Verification items for the finished model (mm, model axes). Coordinates: 2 decimals unless noted, no trailing zeros. Order: outer loops, then holes, each group sorted by start corner. A loop starts at its lowest first (then second) coordinate and runs counter-clockwise, first axis right, second up. Notation, with made-up numbers: (-4.5, 68.5) - (31.5, 68.5) arc R13 cw to (31.5, 93.5) - close; hole circle Ø10 at (42, 48). An arc over 180 degrees is marked (long way). Answer as CSV lines item,"result". Start each with the question number.
1. Section check B-B (z = 1). Record the cut outline in (x, y) (3 decimals), and give its area (3 significant figures).
2. Section check A-A (x = 33.5). Record the cut outline in (y, z) (3 decimals), and give its area (3 significant figures).
3. Section check C-C (x = 25). Record the cut outline in (y, z).
4. Go/stop test with flat-tipped pins: pin 1 (3.5 mm diameter, centred on x = 16.5, y = 16.5, fed in from +Z); pin 2 (2 mm diameter, centred on x = 16.5, y = 33.5, fed in from -Z). Record where each tip stops, or that it passes through.
5. Material ranges on L1, parallel to Y at x = 16.5, z = 1.15 (3 decimals); L2, parallel to Y at x = 26, z = 0.7, recorded low to high. Write a range as [from, to].
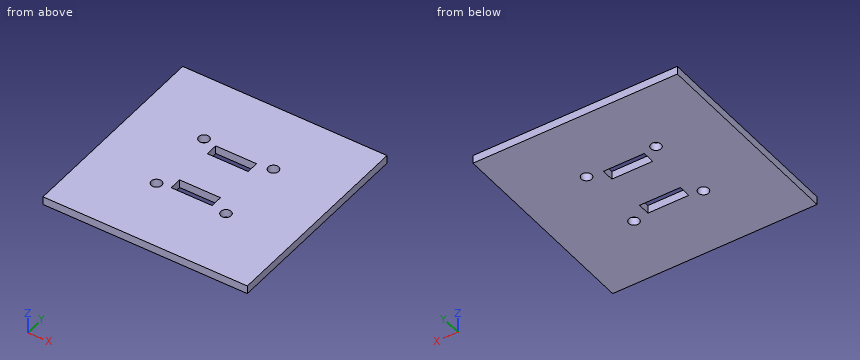
from build123d import *

# Parameters (mm, degrees)
SKETCH1_W           = 50
SKETCH1_H           = 50
BOSS_EXTRUDE1_DEPTH = 2
CUT_EXTRUDE1_REACH  = 72.739
SKETCH3_R           = 1.275
CUT_EXTRUDE2_REACH  = 72.739
SKETCH4_W           = 10
SKETCH4_H           = 3


with BuildPart() as part:
    # Sketch1 → Boss-Extrude1 (new body)
    with BuildSketch(Plane.XY):
        with Locations((25, 25)):
            Rectangle(SKETCH1_W, SKETCH1_H)
    extrude(amount=BOSS_EXTRUDE1_DEPTH)

    # Sketch3 → Cut-Extrude1 (cut, up to next)
    with BuildSketch(Plane.XY.offset(2), mode=Mode.PRIVATE) as cut_extrude1_sk1:
        with Locations((16.5, 33.5)):
            Circle(SKETCH3_R)
    cut_extrude1_tool1 = extrude(cut_extrude1_sk1.sketch, amount=-CUT_EXTRUDE1_REACH, mode=Mode.PRIVATE) & part.part
    # Sketch3 → Cut-Extrude1 (cut, up to next)
    with BuildSketch(Plane.XY.offset(2), mode=Mode.PRIVATE) as cut_extrude1_sk2:
        with Locations((33.5, 33.5)):
            Circle(SKETCH3_R)
    cut_extrude1_tool2 = extrude(cut_extrude1_sk2.sketch, amount=-CUT_EXTRUDE1_REACH, mode=Mode.PRIVATE) & part.part
    # Sketch3 → Cut-Extrude1 (cut, up to next)
    with BuildSketch(Plane.XY.offset(2), mode=Mode.PRIVATE) as cut_extrude1_sk3:
        with Locations((33.5, 16.5)):
            Circle(SKETCH3_R)
    cut_extrude1_tool3 = extrude(cut_extrude1_sk3.sketch, amount=-CUT_EXTRUDE1_REACH, mode=Mode.PRIVATE) & part.part
    # Sketch3 → Cut-Extrude1 (cut, up to next)
    with BuildSketch(Plane.XY.offset(2), mode=Mode.PRIVATE) as cut_extrude1_sk4:
        with Locations((16.5, 16.5)):
            Circle(SKETCH3_R)
    cut_extrude1_tool4 = extrude(cut_extrude1_sk4.sketch, amount=-CUT_EXTRUDE1_REACH, mode=Mode.PRIVATE) & part.part
    add(cut_extrude1_tool1.solids().sort_by_distance((16.5, 33.5, 2))[0], mode=Mode.SUBTRACT)
    add(cut_extrude1_tool2.solids().sort_by_distance((33.5, 33.5, 2))[0], mode=Mode.SUBTRACT)
    add(cut_extrude1_tool3.solids().sort_by_distance((33.5, 16.5, 2))[0], mode=Mode.SUBTRACT)
    add(cut_extrude1_tool4.solids().sort_by_distance((16.5, 16.5, 2))[0], mode=Mode.SUBTRACT)

    # Sketch4 → Cut-Extrude2 (cut, up to next)
    with BuildSketch(Plane.XY.offset(2), mode=Mode.PRIVATE) as cut_extrude2_sk1:
        with Locations((24.7, 31.5)):
            Rectangle(SKETCH4_W, SKETCH4_H)
    cut_extrude2_tool1 = extrude(cut_extrude2_sk1.sketch, amount=-CUT_EXTRUDE2_REACH, mode=Mode.PRIVATE) & part.part
    # Sketch4 → Cut-Extrude2 (cut, up to next)
    with BuildSketch(Plane.XY.offset(2), mode=Mode.PRIVATE) as cut_extrude2_sk2:
        with Locations((24.75, 18.5)):
            Rectangle(SKETCH4_W, SKETCH4_H)
    cut_extrude2_tool2 = extrude(cut_extrude2_sk2.sketch, amount=-CUT_EXTRUDE2_REACH, mode=Mode.PRIVATE) & part.part
    add(cut_extrude2_tool1.solids().sort_by_distance((24.7, 31.5, 2))[0], mode=Mode.SUBTRACT)
    add(cut_extrude2_tool2.solids().sort_by_distance((24.75, 18.5, 2))[0], mode=Mode.SUBTRACT)


solid = part.part
Evaluation:
1,outline,"(0, 0) - (50, 0) - (50, 50) - (0, 50) - close; hole circle Ø2.55 at (16.5, 16.5); hole circle Ø2.55 at (16.5, 33.5); hole (19.7, 30) - (29.7, 30) - (29.7, 33) - (19.7, 33) - close; hole (19.75, 17) - (29.75, 17) - (29.75, 20) - (19.75, 20) - close; hole circle Ø2.55 at (33.5, 16.5); hole circle Ø2.55 at (33.5, 33.5)"
1,area,"2,420 mm²"
2,outline,"(0, 0) - (15.225, 0) - (15.225, 2) - (0, 2) - close; (17.775, 0) - (32.225, 0) - (32.225, 2) - (17.775, 2) - close; (34.775, 0) - (50, 0) - (50, 2) - (34.775, 2) - close"
2,area,"89.8 mm²"
3,outline,"(0, 0) - (17, 0) - (17, 2) - (0, 2) - close; (20, 0) - (30, 0) - (30, 2) - (20, 2) - close; (33, 0) - (50, 0) - (50, 2) - (33, 2) - close"
4,pin 1,"stops at z = 2"
4,pin 2,"passes through"
5,L1,"y = [0, 15.225], [17.775, 32.225], [34.775, 50]"
5,L2,"y = [0, 17], [20, 30], [33, 50]"
